Here's how the part is built. I have some questions about the finished solid (model axes, mm). Face numbers are marked on the shaded views. A direction names the side the tool comes from. Give positions to 0.01 mm unless a question says otherwise; leave off trailing zeros. Write each loop counter-clockwise with the first axis right and the second up, starting at its lowest first coordinate (ties: lowest second). Pieces come first, ordered by that corner, then holes. Notation, with made-up numbers: (23, 51.25) -> (51, 51.25) arc R33 cw to (51, 84.25) -> close; hole circle Ø5 at (61.5, 59). An arc over 180 degrees is marked (long way). Answer as CSV lines item,"result". Start each with the question number.
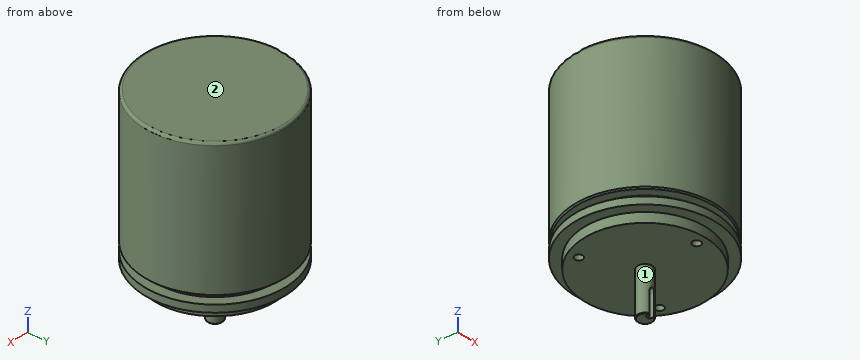
Autodesk Inventor part; units mm, degrees
ref_plane "Work Plane2" through (0, -3, 0) normal (0, -1, 0) x (1, 0, 0)
ref_plane "YZ Plane" through (0, 0, 0) normal (1, 0, 0) x (0, 1, 0)
ref_plane "XZ Plane" through (0, 0, 0) normal (0, 1, 0) x (-1, 0, 0)
sketch "Sketch1" plane through (0, 0, 0) normal (1, 0, 0) x (0, 1, 0)
  line L0 (0, 0) -> (0, 84)
  line L1 (0, 84) -> (29, 84)
  line L2 (29, 84) -> (29, 28)
  line L3 (29, 28) -> (25, 28)
  line L4 (25, 28) -> (25, 25)
  line L5 (25, 25) -> (29, 25)
  line L6 (29, 25) -> (29, 22)
  line L7 (29, 22) -> (25, 22)
  line L8 (25, 22) -> (25, 18)
  line L9 (25, 18) -> (3, 18)
  line L10 (3, 18) -> (3, 0)
  line L11 (3, 0) -> (0, 0)
  dimension "d0" = 84
  dimension "d1" = 29
  dimension "d2" = 56
  dimension "d5" = 4
  dimension "d6" = 3
  dimension "d7" = 4
  dimension "d8" = 3
  dimension "d9" = 4
  dimension "d10" = 4
  dimension "d11" = 22
revolve "Revolution1" add sketch "Sketch1" angle 360 about axis through (0, 0, 0) along (0, 0, 1)
fillet "Fillet1" radius 1 1 edges at (0, -29, 84)
chamfer "Chamfer1" distance 0.5 angle 45 1 edges at (0, -29, 28)
sketch "Sketch2" plane through (0, 0, 18) normal (0, 0, -1) x (-1, 0, 0)
  line L0 (0, 0) -> (0, -21)
  circle A0 centre (0, -21) radius 1
  circle A1 centre (18.1865, 10.5) radius 1
  circle A2 centre (-18.1865, 10.5) radius 1
  dimension "d17" = 21
  dimension "d18" = 2
  dimension "d21" = 360
extrude "Extrusion1" cut sketch "Sketch2" against normal blind 8
hole "Hole1" at (0, -21, 18) direction (0, 0, 1) diameter 3.242 depth 11.8 tip angle 118
hole "Hole2" at (18.1865, 10.5, 18) direction (0, 0, 1) diameter 3.242 depth 11.8 tip angle 118
hole "Hole3" at (-18.1865, 10.5, 18) direction (0, 0, 1) diameter 3.242 depth 11.8 tip angle 118
sketch "Sketch5" plane through (0, 0, 0) normal (0, 0, -1) x (-1, 0, 0)
  point P0 (0, 0)
sketch "Sketch6" plane through (0, 0, 0) normal (0, 0, -1) x (-1, 0, 0)
  line L0 (0, 0) -> (0, -3)
  dimension "d62" = 3
ref_plane "Work Plane2" through (0, -3, 0) normal (0, -1, 0) x (1, 0, 0)
sketch "Sketch7" plane through (0, -3, 0) normal (0, -1, 0) x (1, 0, 0)
  line L0 (-3, 18) -> (-3, 0)
  line L1 (3, 18) -> (3, 0)
  line L2 (-3, 0) -> (3, 0)
  line L3 (-25, 18) -> (25, 18)
  line L4 (-1, 0) -> (1, 0)
  line L5 (1, 0) -> (1, 10)
  line L6 (1, 10) -> (-1, 10)
  line L7 (-1, 10) -> (-1, 0)
  point P0 (0, 0)
  dimension "d63" = 10
  dimension "d64" = 2
  dimension "d66" = 2
extrude "Extrusion3" cut sketch "Sketch7" against normal blind 2 contours L7 L6 L5 L2
chamfer "Chamfer3" distance 0.25 angle 45 2 edges at (2.9568, 0.5073, 0) (-2.9568, 0.5073, 0)
fillet "Fillet2" radius 1 2 edges at (-1, -1.9142, 10) (1, -1.9142, 10)
properties part number "Tachometer"
Item 1: If I drill on line 1 (Z direction, x = -20.5, y = -18); line 2 (Y direction, x = 0, z = 23.5); line 3 (X direction, y = 10.5, z = 25.75), over which ranges is the centre line in solid material (lowest first)? Write a range as [from, to].
Item 2: For the marked faces 1 and 2, which set-ups out of +Z, -Z, +X, -X, +Y, -Y let a thin tool reach every point of the face, with its end or its side?
Item 3: If we section it at D-D (z = 11): Please give me the cut outline in (x, y).
Item 4: I'm going to push flat-ended pins straight in: pin 1 (2 mm diameter, centred on y = 0.5, z = 52.5, fed in from -X); pin 2 (2 mm diameter, centred on y = -2, z = 5.5, fed in from -X); pin 3 (5 mm diameter, centred on x = 0, y = -21, fed in from -Z); pin 4 (17.5 mm diameter, centred on x = -11, y = 1.5, fed in from -Z). Where does each tip first touch, or does it pass through?
Item 5: If we section it at B-B (z = 56): Please give me the cut outline in (x, y), and give its area (3 significant figures).
Item 6: If we section it at A-A (y = 0): Please give me the cut outline in (x, z), and give its area (3 significant figures).
Item 7: If we section it at C-C (z = 23.5): Please give me the cut outline in (x, y).
Final values:
1,line 1,"[22, 25], [28, 84]"
1,line 2,"[-29, -22.62], [-19.38, 29]"
1,line 3,"[-22.69, -19.81], [-16.57, 16.57], [19.81, 22.69]"
2,face 1,"-Z"
2,face 2,"+Z, +X, -X, +Y, -Y"
3,outline,"circle Ø6 at (0, 0)"
4,pin 1,"x = -29"
4,pin 2,"x = -2.83"
4,pin 3,"z = 18"
4,pin 4,"z = 0"
5,outline,"circle Ø58 at (0, 0)"
5,area,"2,640 mm2"
6,outline,"(-29, 22) -> (-25, 22) -> (-25, 18) -> (-3, 18) -> (-3, 0.25) -> (-2.75, 0) -> (2.75, 0) -> (3, 0.25) -> (3, 18) -> (25, 18) -> (25, 22) -> (29, 22) -> (29, 25) -> (25, 25) -> (25, 28) -> (28.5, 28) -> (29, 28.5) -> (29, 83) arc R1 ccw to (28, 84) -> (-28, 84) arc R1 ccw to (-29, 83) -> (-29, 28.5) -> (-28.5, 28) -> (-25, 28) -> (-25, 25) -> (-29, 25) -> close"
6,area,"3,880 mm2"
7,outline,"circle Ø58 at (0, 0); hole circle Ø3.24 at (-18.19, 10.5); hole circle Ø3.24 at (0, -21); hole circle Ø3.24 at (18.19, 10.5)"
